from build123d import *

# Parameters (mm, degrees)
SKETCH1_W                                           = 150
SKETCH1_H                                           = 150
BOSS_EXTRUDE1_DEPTH                                 = 5
CBORE_FOR_M5_HEX_SOCKET_HEAD_CAP_SCREW1_D           = 5.5
CBORE_FOR_M5_HEX_SOCKET_HEAD_CAP_SCREW1_CBORE_D     = 10
CBORE_FOR_M5_HEX_SOCKET_HEAD_CAP_SCREW1_CBORE_DEPTH = 5.5
F_11_0_11_DIAMETER_HOLE1_D                          = 11
SKETCH6_R                                           = 12
CUT_EXTRUDE1_DEPTH                                  = 2.5
FILLET2_R                                           = 0.3
BOSS_EXTRUDE2_DEPTH                                 = 10
FILLET3_R                                           = 5
F_4_5_4_5_DIAMETER_HOLE1_D                          = 4.5
FILLET4_R                                           = 2
M3_TAPPED_HOLE1_D                                   = 2.5
CHAMFER1_SIZE                                       = 0.5


with BuildPart() as part:
    # Sketch1 → Boss-Extrude1 (new, symmetric)
    with BuildSketch(Plane(origin=(0, 0, 0), x_dir=(1, 0, 0), z_dir=(0, 1, 0))):
        Rectangle(SKETCH1_W, SKETCH1_H)
    extrude(amount=BOSS_EXTRUDE1_DEPTH, both=True)

    # CBORE for M5 Hex Socket Head Cap Screw1 (through all)
    with Locations(Plane(origin=(0, -5, 0), x_dir=(-1, 0, 0), z_dir=(0, -1, 0))):
        with Locations((-65, -65), (-65, -25), (-65, 25), (-65, 65), (65, -65), (65, -25), (65, 25), (65, 65)):
            CounterBoreHole(CBORE_FOR_M5_HEX_SOCKET_HEAD_CAP_SCREW1_D / 2, CBORE_FOR_M5_HEX_SOCKET_HEAD_CAP_SCREW1_CBORE_D / 2, CBORE_FOR_M5_HEX_SOCKET_HEAD_CAP_SCREW1_CBORE_DEPTH)

    # Ø11.0 (11) Diameter Hole1 (through all)
    with Locations(Plane(origin=(0, -5, 0), x_dir=(-1, 0, 0), z_dir=(0, -1, 0))):
        with Locations((0, 0)):
            Hole(F_11_0_11_DIAMETER_HOLE1_D / 2)

    # Sketch6 → Cut-Extrude1 (cut)
    with BuildSketch(Plane.XZ.offset(-5)):
        with Locations(Location((0, 0, 0), (0, 0, 270))):
            Circle(SKETCH6_R)
    extrude(amount=CUT_EXTRUDE1_DEPTH, mode=Mode.SUBTRACT)

    # Fillet2
    fillet2_edges = [part.edges().sort_by_distance(p)[0] for p in [
        (0, 2.5, 12),
    ]]
    fillet(fillet2_edges, radius=FILLET2_R)

    # Sketch7 → Boss-Extrude2 (add)
    with BuildSketch(Plane(origin=(0, 5, 0), x_dir=(1, 0, 0), z_dir=(0, 1, 0))):
        Polygon((-75, 25), (-75, -25), (-120, -15), (-120, 15), align=None)
    extrude(amount=-BOSS_EXTRUDE2_DEPTH)

    # Fillet3
    fillet3_edges = [part.edges().sort_by_distance(p)[0] for p in [
        (-75, 0, -25),
        (-75, 0, 25),
    ]]
    fillet(fillet3_edges, radius=FILLET3_R)

    # Ø4.5 (4.5) Diameter Hole1 (through all)
    with Locations(Plane(origin=(0, 5, 0), x_dir=(1, 0, 0), z_dir=(0, 1, 0))):
        with Locations((-110, 10), (-110, -10)):
            Hole(F_4_5_4_5_DIAMETER_HOLE1_D / 2)

    # Fillet4
    fillet4_edges = [part.edges().sort_by_distance(p)[0] for p in [
        (-120, 0, -15),
        (-120, 0, 15),
    ]]
    fillet(fillet4_edges, radius=FILLET4_R)

    # M3 Tapped Hole1 (through all)
    with Locations(Plane(origin=(0, 5, 0), x_dir=(1, 0, 0), z_dir=(0, 1, 0))):
        with Locations((-25, -63), (25, -63)):
            Hole(M3_TAPPED_HOLE1_D / 2)

    # Chamfer1
    chamfer1_edges = [part.edges().sort_by_distance(p)[0] for p in [
        (0, 5, 12),
    ]]
    chamfer(chamfer1_edges, length=CHAMFER1_SIZE)


solid = part.part
The model under review builds one solid part; all positions refer to its coordinate system, in mm. A direction names the side the tool comes from. Give positions to 0.01 mm unless a question says otherwise; leave off trailing zeros. Write each loop counter-clockwise with the first axis right and the second up, starting at its lowest first coordinate (ties: lowest second). Pieces come first, ordered by that corner, then holes.
1. Add section C-C, the plane y = -2. Count the separate pieces of the cut face and the enclosed holes in it, plus the area to 3 significant figures.
2. Draft analysis for pull direction X (two halves, no side actions). For faces 3 (the cylindrical face through (-1.19, -1.2, 5.37)), 4 (the flat face through (-98.951, 0.07, -19.678)), 5 (the flat face through (75, 0, 1)), state which applies: +X half, -X half, draft (parallel to the pull), parting line (faces both ways), or undercut.
3. Add section B-B, the plane z = 0. Write out the cut boundary in (x, y), plus the area to 3 significant figures.
4. Add section A-A, the plane x = 0. Write out the cut boundary in (y, z), plus the area to 3 significant figures.
5. Add section D-D, the plane z = -65. Write out the cut boundary in (x, y).
6. Tool access review of faces 1 (the cylindrical face through (62.253, 2.781, 24.879)), 2 (the cylindrical face through (-68, -2, -69)): name each direction out of +Z, -Z, +X, -X, +Y, -Y from which nothing blocks a thin tool from reaching the whole face with its end or side.
7. Wall thickness on L1, parallel to Z at x = -65, y = 2.4; L2, parallel to X at y = 1.6, z = 65; L3, parallel to X at y = -1.8, z = 65: over which ranges is each line inside the solid? List them lowest first.
8. For P1, Ø7, axis at x = 4, z = 5, coming from the +Y side; P2, Ø4, axis at x = -90.5, y = 1, coming from the -Z side; P3, Ø9, axis at x = -65, z = 65, coming from the -Y side, all flat-tipped, find the tip position at first contact; note any pin that passes through.
Worked answers:
1. separate pieces: 1
1. enclosed holes: 13
1. area: 23,500 mm2
2. face 3: undercut
2. face 4: -X half
2. face 5: +X half
3. outline: (-120, -5) - (-5.5, -5) - (-5.5, 2.5) - (-11.7, 2.5) arc R0.3 cw to (-12, 2.8) - (-12, 4.5) - (-12.5, 5) - (-120, 5) - close; (5.5, -5) - (75, -5) - (75, 5) - (12.5, 5) - (12, 4.5) - (12, 2.8) arc R0.3 cw to (11.7, 2.5) - (5.5, 2.5) - close
3. area: 1,810 mm2
4. outline: (-5, -75) - (5, -75) - (5, -12.5) - (4.5, -12) - (2.8, -12) arc R0.3 cw to (2.5, -11.7) - (2.5, -5.5) - (-5, -5.5) - close; (-5, 5.5) - (2.5, 5.5) - (2.5, 11.7) arc R0.3 cw to (2.8, 12) - (4.5, 12) - (5, 12.5) - (5, 75) - (-5, 75) - close
4. area: 1,360 mm2
5. outline: (-75, -5) - (-70, -5) - (-70, 0.5) - (-67.75, 0.5) - (-67.75, 5) - (-75, 5) - close; (-62.25, 0.5) - (-60, 0.5) - (-60, -5) - (60, -5) - (60, 0.5) - (62.25, 0.5) - (62.25, 5) - (-62.25, 5) - close; (67.75, 0.5) - (70, 0.5) - (70, -5) - (75, -5) - (75, 5) - (67.75, 5) - close
6. face 1: +Y, -Y
6. face 2: -Y
7. L1: z = -75 to -67.75, -62.25 to -27.75, -22.25 to 22.25, 27.75 to 62.25, 67.75 to 75
7. L2: x = -75 to -67.75, -62.25 to 62.25, 67.75 to 75
7. L3: x = -75 to -70, -60 to 60, 70 to 75
8. P1: stops at y = 2.5
8. P2: stops at z = -22
8. P3: stops at y = 0.5
